```python
from build123d import *

# Parameters (mm, degrees)
SKETCH_1_R      = 2.95
SKETCH_1_R_2    = 2
EXTRUDE_1_DEPTH = 8.5
EXTRUDE_START   = 0.75
SKETCH_2_R      = 3.55
SKETCH_2_R_2    = 2
EXTRUDE_2_DEPTH = 0.75
SKETCH_3_W      = 0.5
SKETCH_3_H      = 1.5
CHAMFER_1_SIZE  = 0.4


with BuildPart() as part:
    # 草图1 → 凸台-拉伸1 (new body)
    with BuildSketch(Plane(origin=(0, 0, 0), x_dir=(1, 0, 0), z_dir=(0, 1, 0))):
        with Locations(Location((0, 0, 0), (0, 0, 270))):
            Circle(SKETCH_1_R)
        with Locations(Location((0, 0, 0), (0, 0, 270))):
            Circle(SKETCH_1_R_2, mode=Mode.SUBTRACT)
    extrude(amount=-EXTRUDE_1_DEPTH)

    # 草图2 → 凸台-拉伸2 (add)
    with BuildSketch(Plane(origin=(0, 0, 0), x_dir=(1, 0, 0), z_dir=(0, 1, 0)).offset(EXTRUDE_START)):
        with Locations(Location((0, 0, 0), (0, 0, 270))):
            Circle(SKETCH_2_R)
        with Locations(Location((0, 0, 0), (0, 0, 270))):
            Circle(SKETCH_2_R_2, mode=Mode.SUBTRACT)
    extrude(amount=-EXTRUDE_2_DEPTH)

    # 草图3 → 切除-旋转1 (revolve, cut)
    with BuildSketch(Plane(origin=(0, 0, 0), x_dir=(0, 0, -1), z_dir=(1, 0, 0))):
        with Locations((-2.7, -7.25)):
            Rectangle(SKETCH_3_W, SKETCH_3_H)
    revolve(axis=Axis((0, 0, 0), (0, -1, 0)), mode=Mode.SUBTRACT)

    # 倒角1
    chamfer_1_edges = [part.edges().sort_by_distance(p)[0] for p in [
        (0, 0.75, -2),
        (0, -6.5, -2.95),
        (0, -8.5, -2.95),
    ]]
    chamfer(chamfer_1_edges, length=CHAMFER_1_SIZE)


solid = part.part
```
Work out the finished part from the listing and answer in its coordinate system (mm). A direction names the side the tool comes from. Give positions to 0.01 mm unless a question says otherwise; leave off trailing zeros. Write each loop counter-clockwise with the first axis right and the second up, starting at its lowest first coordinate (ties: lowest second). Pieces come first, ordered by that corner, then holes. Notation, with made-up numbers: (20, 9.5) -> (72, 9.5) arc R26 cw to (72, 38.5) -> close; hole circle Ø3 at (35.25, 46). An arc over 180 degrees is marked (long way). Write item = value, one per line.
Q1. Consider line 1 along X through (y, z) = (-1.75, 0); line 2 along Y through (x, z) = (2, 1.5); line 3 along Y through (x, z) = (1.5, -2.25). Determine where each line is inside the solid, lowest interval first.
Computed values:
line_1 = -2.95 to -2, 2 to 2.95
line_2 = -8.5 to -8, -6.5 to 0.75
line_3 = -8.35 to -8, -6.35 to 0.75
Q2. Section D-D on y = -5.75 is taken. Determine the outline of the cut face in (x, z), and give its area (3 significant figures).
Computed values:
outline = circle Ø5.9 at (0, 0); hole circle Ø4 at (0, 0)
area = 14.8 mm^2
Q3. Flat-ended cylindrical pins translate along their axes: pin 1 Ø2 at (x, y) = (0, -3.5) entering from -Z; pin 2 Ø2 at (x, y) = (-2, -1.5) entering from -Z; pin 3 Ø1 at (x, y) = (3, -3) entering from +Z. Find the tip coordinate at first contact, or state that the pin passes through.
Computed values:
pin_1 = -2.95
pin_2 = -2.78
pin_3 = 1.57
Q4. A tool of negligible diameter and unlimited length cuts with its end or side. For faces 1 (the flat face through (3, 0, 1)), 2 (the cylindrical face through (2.4, -7.2, -0.5)), 3 (the cylindrical face through (3, 0.4, 1.9)), from which of +Z, -Z, +X, -X, +Y, -Y can it reach the whole face along a straight path? Write none if from no direction.
Computed values:
face_1 = -Y
face_2 = none
face_3 = +Y, -Y
Q5. Section A-A on x = 0 is taken. Determine the outline of the cut face in (y, z).
Computed values:
outline = (-8.5, -2.55) -> (-8.1, -2.95) -> (-8, -2.95) -> (-8, -2.45) -> (-6.5, -2.45) -> (-6.5, -2.55) -> (-6.1, -2.95) -> (0, -2.95) -> (0, -3.55) -> (0.75, -3.55) -> (0.75, -2.4) -> (0.35, -2) -> (-8.5, -2) -> close; (-8.5, 2) -> (0.35, 2) -> (0.75, 2.4) -> (0.75, 3.55) -> (0, 3.55) -> (0, 2.95) -> (-6.1, 2.95) -> (-6.5, 2.55) -> (-6.5, 2.45) -> (-8, 2.45) -> (-8, 2.95) -> (-8.1, 2.95) -> (-8.5, 2.55) -> close
Q6. For a pull along Z with two mould halves and no side action, classify faces 4 (the flat face through (-1, -8.5, -2)), 5 (the cylindrical face through (-2.88, -3.01, -0.64)), 6 (the cylindrical face through (-2, -4, 0)) as pulls with the +Z half, pulls with the -Z half, needs draft (parallel to the pull), parting line crosses it, or undercut.
Computed values:
face_4 = needs draft
face_5 = parting line crosses it
face_6 = undercut
Q7. Section B-B on z = 0 is taken. Determine the outline of the cut face in (x, y).
Computed values:
outline = (-3.55, 0) -> (-2.95, 0) -> (-2.95, -6.1) -> (-2.55, -6.5) -> (-2.45, -6.5) -> (-2.45, -8) -> (-2.95, -8) -> (-2.95, -8.1) -> (-2.55, -8.5) -> (-2, -8.5) -> (-2, 0.35) -> (-2.4, 0.75) -> (-3.55, 0.75) -> close; (2, -8.5) -> (2.55, -8.5) -> (2.95, -8.1) -> (2.95, -8) -> (2.45, -8) -> (2.45, -6.5) -> (2.55, -6.5) -> (2.95, -6.1) -> (2.95, 0) -> (3.55, 0) -> (3.55, 0.75) -> (2.4, 0.75) -> (2, 0.35) -> close
Q8. Section C-C on y = -6.75 is taken. Determine the outline of the cut face in (x, z).
Computed values:
outline = circle Ø4.9 at (0, 0); hole circle Ø4 at (0, 0)
